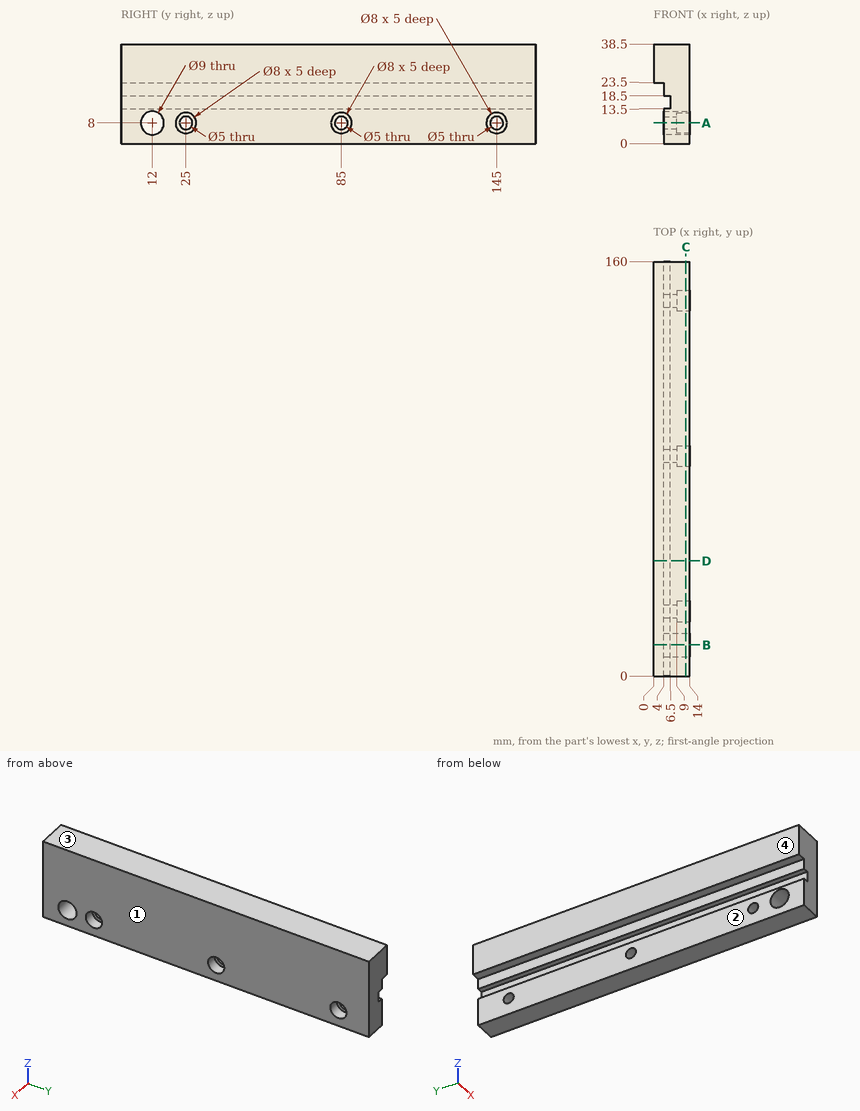
Source: three-view drawing plus pictorial views. Frame: mm from the lowest corner of the part. A direction names the side the tool comes from. Coordinates: 2 decimals unless noted, no trailing zeros. Loops run counter-clockwise (first coordinate to the right, second up) from the corner with the lowest first, then second, coordinate; pieces in that order, holes last. Notation, with made-up numbers: (86, 61.25) -> (114, 61.25) arc R29 ccw to (114, 95.25) -> close; hole circle Ø8 at (-4, 70.25). An arc over 180 degrees is marked (long way). Answer in a Markdown table with one row per item. Add a question column.
Q1. Pull-direction query (Z, two-part tool) for the marked faces 3 and 4; classes: pulls with the +Z half, pulls with the -Z half, needs draft (parallel to the pull), parting line crosses it, or undercut.
Q2. Reachability of the marked faces 1 and 2 from +Z, -Z, +X, -X, +Y, -Y: full face, straight path, thin tool, end or side. Return the list, or none.
Q3. Section B-B on y = 12. Return the cut outline in (x, z).
Q4. Section D-D on y = 44.5. Return the cut outline in (x, z).
Q5. Section C-C on x = 12.5. Return the cut outline in (y, z).
Q6. Ray query, line 1 along Y through (x, z) = (7.35, 8); line 2 along Y through (x, z) = (12.75, 8); line 3 along Z through (x, y) = (3.5, 27.5). Return the intervals inside material, ascending.
Q7. Contact query for flat-ended pins moving along their axis: pin 1 Ø14.5 at (y, z) = (12, 8) entering from -X; pin 2 Ø1.5 at (y, z) = (92, 15.5) entering from -X. Output: stop coordinate, or through.
Q8. Section A-A on z = 8. Give the number of separate pieces and of enclosed holes in the cut face, and give its area (4 significant figures).
Computed values:
| question | item | result |
|---|---|---|
| 1 | face 3 | pulls with the +Z half |
| 1 | face 4 | needs draft |
| 2 | face 1 | +Z, -Z, +X, +Y, -Y |
| 2 | face 2 | -Z, -X, +Y, -Y |
| 3 | outline | (0, 23.5) -> (4, 23.5) -> (4, 18.5) -> (6.5, 18.5) -> (6.5, 13.5) -> (4, 13.5) -> (4, 12.5) -> (14, 12.5) -> (14, 38.5) -> (0, 38.5) -> close; (4, 0) -> (14, 0) -> (14, 3.5) -> (4, 3.5) -> close |
| 4 | outline | (0, 23.5) -> (4, 23.5) -> (4, 18.5) -> (6.5, 18.5) -> (6.5, 13.5) -> (4, 13.5) -> (4, 0) -> (14, 0) -> (14, 38.5) -> (0, 38.5) -> close |
| 5 | outline | (0, 0) -> (160, 0) -> (160, 38.5) -> (0, 38.5) -> close; hole circle Ø9 at (12, 8); hole circle Ø8 at (25, 8); hole circle Ø8 at (85, 8); hole circle Ø8 at (145, 8) |
| 6 | line 1 | y = 0 to 7.5, 16.5 to 22.5, 27.5 to 82.5, 87.5 to 142.5, 147.5 to 160 |
| 6 | line 2 | y = 0 to 7.5, 16.5 to 21, 29 to 81, 89 to 141, 149 to 160 |
| 6 | line 3 | z = 23.5 to 38.5 |
| 7 | pin 1 | stops at x = 4 |
| 7 | pin 2 | stops at x = 6.5 |
| 8 | separate pieces | 5 |
| 8 | enclosed holes | 0 |
| 8 | area | 1,315 mm^2 |
